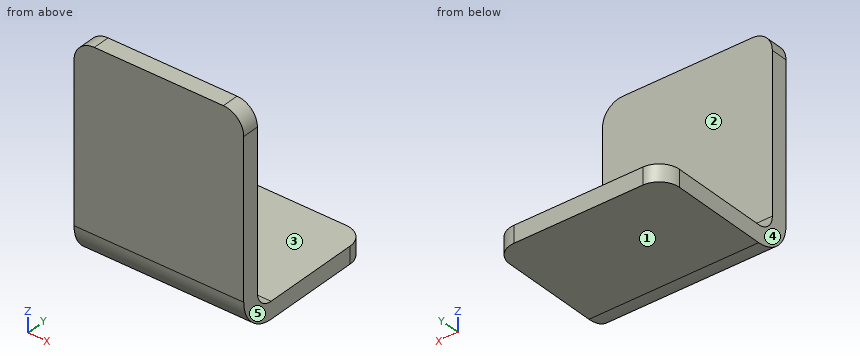
Autodesk Inventor part; units mm, degrees
ref_plane "YZ Plane" through (0, 0, 0) normal (1, 0, 0) x (0, 1, 0)
ref_plane "XZ Plane" through (0, 0, 0) normal (0, 1, 0) x (-1, 0, 0)
ref_plane "XY Plane" through (0, 0, 0) normal (0, 0, 1) x (1, 0, 0)
sketch "Schizzo1" plane through (0, 0, 0) normal (0, 0, 1) x (1, 0, 0)
  line L0 (-25, 17.5) -> (25, 17.5)
  line L1 (25, 17.5) -> (25, -17.5)
  line L2 (25, -17.5) -> (-25, -17.5)
  line L3 (-25, -17.5) -> (-25, 17.5)
  line L4 (-25, 17.5) -> (25, -17.5) construction
  line L5 (25, 17.5) -> (-25, -17.5) construction
  point P0 (0, 0)
  dimension "d0" = 50
  dimension "d1" = 35
extrude "Piano1" add sketch "Schizzo1" along normal blind 5
sketch "Schizzo2" plane through (25, -22.5, 10) normal (0, -1, 0) x (1, 0, 0)
  line L0 (-50, 0) -> (0, 0)
  line L1 (0, 0) -> (0, 52)
  line L2 (0, 52) -> (-50, 52)
  line L3 (-50, 52) -> (-50, 0)
edge flange "Flangia1" height 62 angle 90 thickness 5 bend radius 5 thickness toward (0, -1, 0) relief tear relief width 5 relief depth 2.5 edges at (0, -17.5, 5) wall of the first edge with corners at (-25, -22.5, 10) (25, -22.5, 10) (25, -22.5, 62) (-25, -22.5, 62)
bend "Piega (Bend)1"
corner "Angolo1"
fillet "Arrotondamento angolo1" radius 6 4 edges at (-25, 17.5, 2.5) (25, 17.5, 2.5) (25, -25, 62) (-25, -25, 62)
equation "\"d2\" = Spessore"
equation "\"d3\" = LarghezzaScaricoPiega"
equation "\"d4\" = ProfonditàScaricoPiega"
equation "\"d5\" = ResiduoMinimo"
equation "\"d6\" = RaggioTransizione"
equation "\"d9\" = RaggioPiega"
equation "\"d10\" = DimensioniScaricoAngolo"
equation "\"d11\" = DimensioneGioco"
equation "\"d12\" = Dimensione_raggio_Jacobi"
equation "\"RaggioPiega\" = Spessore"
equation "\"LarghezzaScaricoPiega\" = Spessore"
equation "\"ProfonditàScaricoPiega\" = 0.5 * Spessore"
equation "\"RaggioTransizione\" = RaggioPiega"
equation "\"Dimensione_raggio_Jacobi\" = RaggioPiega"
equation "\"DimensioneGioco\" = Spessore"
properties part number "Lamiera 10mm supporto asse"
Could you check a few things on this model? Use its own coordinates, in mm. Face numbers are marked on the shaded views. A direction names the side the tool comes from. Give positions to 0.01 mm unless a question says otherwise; leave off trailing zeros. Order: outer loops, then holes, each group sorted by start corner. A loop starts at its lowest first (then second) coordinate and runs counter-clockwise, first axis right, second up. Notation, with made-up numbers: (15.5, -11) -> (60.5, -11) arc R6 cw to (60.5, -2) -> close; hole circle Ø9 at (23, 76). An arc over 180 degrees is marked (long way). Answer in a Markdown table with one row per item. Add a question column.
Item 1: Imagine slicing it at A-A (x = 3). List the corners of the cut face in (y, z) for me.
Item 2: For the marked faces 1 and 2, which set-ups out of +Z, -Z, +X, -X, +Y, -Y let a thin tool reach every point of the face, with its end or its side?
Item 3: Imagine slicing it at C-C (y = 7.5). List the corners of the cut face in (x, z) for me, and give its area (3 significant figures).
Item 4: Please list where these lines run through material, in increasing order: probe 1 along Y at (x, z) = (-16, 18); probe 2 along Z at (x, y) = (-3.5, 13); probe 3 along Z at (x, y) = (7, -18.5).
Item 5: Imagine slicing it at B-B (z = 52). List the corners of the cut face in (x, y) for me.
Item 6: I'm going to push flat-ended pins straight in: P1, Ø10.5, axis at x = 9, y = 1, coming from the +Z side; P2, Ø25, axis at x = 1.5, z = 34, coming from the +Y side; P3, Ø3, axis at x = 2.5, z = 9, coming from the +Y side. Where does each tip first touch, or does it pass through?
Item 7: We'd pull the mould along X, two halves only. Please class the marked faces 3, 4 and 5: pulls with the +X half, pulls with the -X half, needs draft (parallel to the pull), parting line crosses it, or undercut.
Item 8: Imagine slicing it at D-D (x = 21). List the corners of the cut face in (y, z) for me, and give its area (3 significant figures).
Result:
| question | item | result |
|---|---|---|
| 1 | outline | (-27.5, 10) arc R10 ccw to (-17.5, 0) -> (17.5, 0) -> (17.5, 5) -> (-17.5, 5) arc R5 cw to (-22.5, 10) -> (-22.5, 62) -> (-27.5, 62) -> close |
| 2 | face 1 | -Z, +X, -X, +Y, -Y |
| 2 | face 2 | +Z, +X, -X, +Y |
| 3 | outline | (-25, 0) -> (25, 0) -> (25, 5) -> (-25, 5) -> close |
| 3 | area | 250 mm2 |
| 4 | probe 1 | -27.5 to -22.5 |
| 4 | probe 2 | 0 to 5 |
| 4 | probe 3 | 0.05 to 5.1 |
| 5 | outline | (-25, -27.5) -> (25, -27.5) -> (25, -22.5) -> (-25, -22.5) -> close |
| 6 | P1 | z = 5 |
| 6 | P2 | y = -22.5 |
| 6 | P3 | y = -21.83 |
| 7 | face 3 | needs draft |
| 7 | face 4 | pulls with the -X half |
| 7 | face 5 | pulls with the +X half |
| 8 | outline | (-27.5, 10) arc R10 ccw to (-17.5, 0) -> (17.16, 0) -> (17.16, 5) -> (-17.5, 5) arc R5 cw to (-22.5, 10) -> (-22.5, 61.66) -> (-27.5, 61.66) -> close |
| 8 | area | 490 mm2 |
